```python
from build123d import *

# Parameters (mm, degrees)
F2_R = 0.99999
F3_R = 0.5


# Not quite as in the source:
# - a fillet or chamfer is up to 0.001 mm smaller than in the source, because OpenCascade refuses the exact size


with BuildPart() as f1:
    # F0 (on Front) → F1 (revolve)
    with BuildSketch(Plane.XZ):
        Polygon((19.1826918498, 16.5195801589), (-8.8173081502, 16.5195801589), (-8.8173081502, -3.4804198411), (-6.8173081502, -3.4804198411), (-6.8173081502, 14.5195801589), (19.1826918498, 14.5195801589), align=None)
    revolve(axis=Axis((19.1826918498, 0, 15.5195801589), (0, 0, -1)))

    # F2 (radius 1 in the source; OpenCascade refuses exactly that, so slightly less here)
    f2_edges = [f1.edges().sort_by_distance(p)[0] for p in [
        (47.182692, 0, -3.48042),
        (45.182692, 0, -3.48042),
    ]]
    fillet(f2_edges, radius=F2_R)

    # F3
    f3_edges = [f1.edges().sort_by_distance(p)[0] for p in [
        (45.182692, 0, 14.51958),
    ]]
    fillet(f3_edges, radius=F3_R)


solid = f1.part
```
Check sheet for the modelled part. Datum: model origin and axes. Units: mm. Round coordinates to 2 decimals unless told otherwise and drop trailing zeros. Order: outer loops, then holes, each group sorted by start corner. A loop starts at its lowest first (then second) coordinate and runs counter-clockwise, first axis right, second up. Notation, with made-up numbers: (-30.75, 3) - (21.25, 3) arc R18 cw to (21.25, 36) - close; hole circle Ø9 at (-35.75, -30.5). An arc over 180 degrees is marked (long way). Write item = value, one per line.
Q1. Draft check along Y on faces 1 (the face through (-7.524, 8.41, 6.887)), 2 (the face through (20, 0, 14.52)), 3 (the face through (19, 0, 16.52)). Enter one of: pulls with the +Y half, pulls with the -Y half, needs draft (parallel to the pull), parting line crosses it, or undercut.
Computed:
face_1 = parting line crosses it
face_2 = undercut
face_3 = needs draft
Q2. Section check A-A (z = 1.5). Record the boundary of the cut face in (x, y), and give its area (3 significant figures).
Computed:
outline = circle Ø56 at (19.18, 0); hole circle Ø52 at (19.18, 0)
area = 339 mm^2
Q3. Go/stop test with flat-tipped pins: pin 1 (2 mm diameter, centred on x = 23, y = -3.5, fed in from -Z); pin 2 (3 mm diameter, centred on y = 20, z = 13.5, fed in from -X); pin 3 (1.5 mm diameter, centred on x = -2.5, z = 6, fed in from +Y). Record where each tip stops, or that it passes through.
Computed:
pin_1 = 14.52
pin_2 = -1.84
pin_3 = 18.6
Q4. Thickness scan on line 1 along Z through (x, y) = (18.5, -22.5); line 2 along X through (y, z) = (-12, 1.25); line 3 along X through (y, z) = (-11.5, 3.5). Record the ranges inside material, lowest first.
Computed:
line_1 = 14.52 to 16.52
line_2 = -6.12 to -3.88, 42.25 to 44.48
line_3 = -6.35 to -4.14, 42.5 to 44.71
